Part print with two shaded views. Sizes in mm from the minimum x, y, z corner. Round coordinates to 2 decimals unless told otherwise and drop trailing zeros. Loops run counter-clockwise (first coordinate to the right, second up) from the corner with the lowest first, then second, coordinate; pieces in that order, holes last. Notation, with made-up numbers: (48.25, 38.25) -> (77.25, 38.25) arc R15 ccw to (77.25, 47.25) -> close; hole circle Ø2 at (83, 69.25). An arc over 180 degrees is marked (long way). Use a Markdown table: item, result. Add a question column.
Item 1: Cut at D-D, the plane x = 75. List the corners of the cut face in (y, z), plus the area to 3 significant figures.
Item 2: Cut at A-A, the plane y = 6.5. State how many separate pieces and enclosed holes the cut face has, plus the area to 3 significant figures.
Item 3: Cut at B-B, the plane x = 50. List the corners of the cut face in (y, z).
Item 4: Flat gauge pins, fed straight in: pin 1 (1.5 mm diameter, centred on y = 11, z = 21.5, fed in from -X); pin 2 (4 mm diameter, centred on y = 8.5, z = 30.5, fed in from +X); pin 3 (1.5 mm diameter, centred on y = 7.5, z = 13.5, fed in from +X); pin 4 (2.5 mm diameter, centred on x = 50, z = 95, fed in from +Y). Where does each tip first touch, or does it go through?
Item 5: Probe line 1 (X direction, y = 10.25, z = 50); line 2 (Z direction, x = 26.5, y = 12.75); line 3 (X direction, y = 13.75, z = 34.5). List the from-to ranges inside material, lowest first. Write a range as [from, to].
Item 6: Cut at C-C, the plane z = 5. List the corners of the cut face in (x, y), plus the area to 3 significant figures.
Item 7: Two-plate mould, pull along X, no slides. Class the marked faces 1, 2 and 3: pulls with the +X half, pulls with the -X half, needs draft (parallel to the pull), parting line crosses it, or undercut.
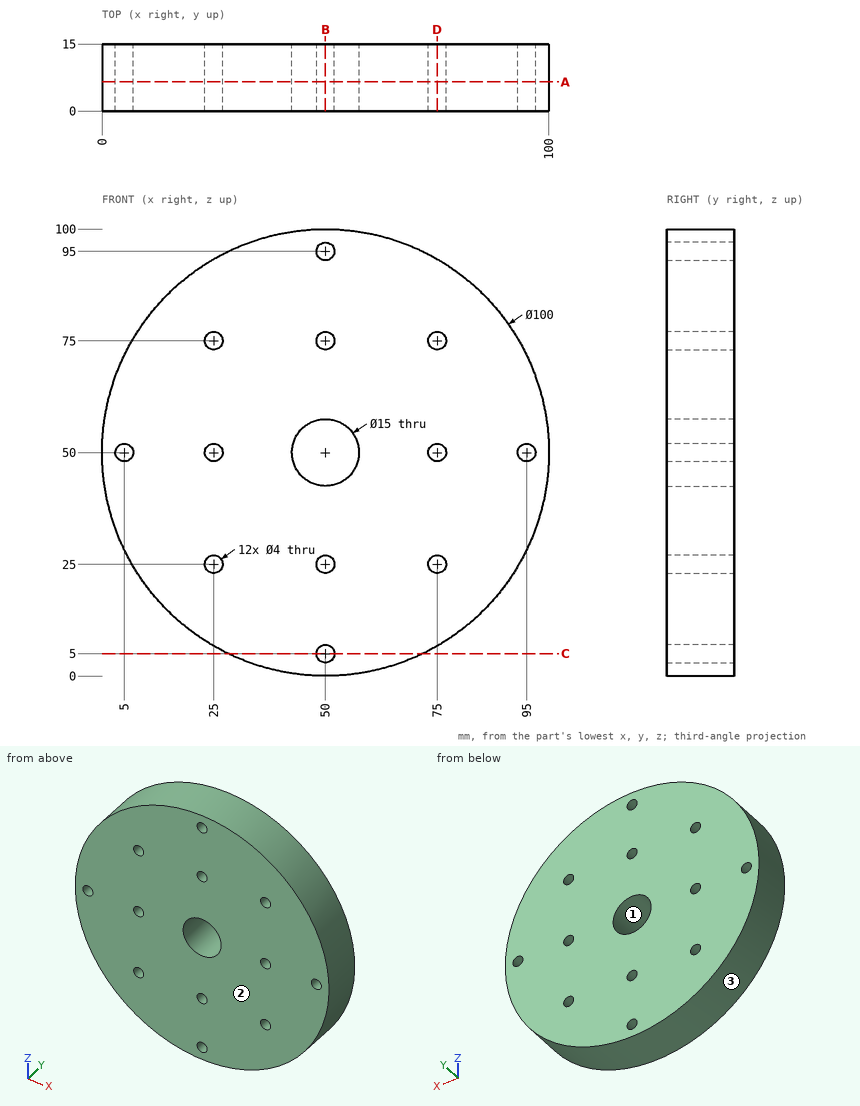
A:
| question | item | result |
|---|---|---|
| 1 | outline | (0, 6.7) -> (15, 6.7) -> (15, 23) -> (0, 23) -> close; (0, 27) -> (15, 27) -> (15, 48) -> (0, 48) -> close; (0, 52) -> (15, 52) -> (15, 73) -> (0, 73) -> close; (0, 77) -> (15, 77) -> (15, 93.3) -> (0, 93.3) -> close |
| 1 | area | 1,120 mm^2 |
| 2 | separate pieces | 1 |
| 2 | enclosed holes | 13 |
| 2 | area | 7,530 mm^2 |
| 3 | outline | (0, 0) -> (15, 0) -> (15, 3) -> (0, 3) -> close; (0, 7) -> (15, 7) -> (15, 23) -> (0, 23) -> close; (0, 27) -> (15, 27) -> (15, 42.5) -> (0, 42.5) -> close; (0, 57.5) -> (15, 57.5) -> (15, 73) -> (0, 73) -> close; (0, 77) -> (15, 77) -> (15, 93) -> (0, 93) -> close; (0, 97) -> (15, 97) -> (15, 100) -> (0, 100) -> close |
| 4 | pin 1 | stops at x = 8.41 |
| 4 | pin 2 | stops at x = 96.84 |
| 4 | pin 3 | stops at x = 84.96 |
| 4 | pin 4 | passes through |
| 5 | line 1 | x = [0, 3], [7, 23], [27, 42.5], [57.5, 73], [77, 93], [97, 100] |
| 5 | line 2 | z = [5.87, 23.68], [26.32, 48.68], [51.32, 73.68], [76.32, 94.13] |
| 5 | line 3 | x = [2.46, 97.54] |
| 6 | outline | (28.21, 0) -> (48, 0) -> (48, 15) -> (28.21, 15) -> close; (52, 0) -> (71.79, 0) -> (71.79, 15) -> (52, 15) -> close |
| 6 | area | 594 mm^2 |
| 7 | face 1 | undercut |
| 7 | face 2 | needs draft |
| 7 | face 3 | parting line crosses it |
